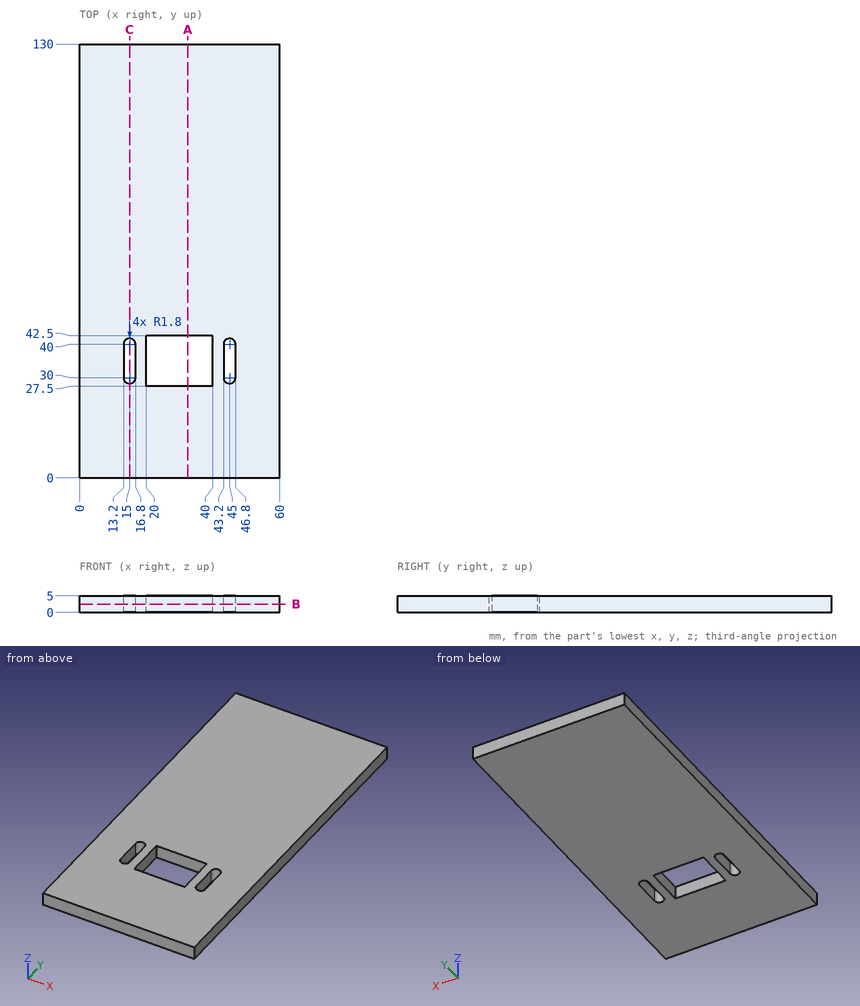
Source: three-view drawing plus pictorial views. Frame: mm from the lowest corner of the part. Give positions to 0.01 mm unless a question says otherwise; leave off trailing zeros. Loops run counter-clockwise (first coordinate to the right, second up) from the corner with the lowest first, then second, coordinate; pieces in that order, holes last.
1) Line query: L1, parallel to X at y = 37, z = 0.25; L2, parallel to Y at x = 31.5, z = 1.2. Output: solid intervals per line, ascending.
A:
L1: x = 0 to 13.2, 16.8 to 20, 40 to 43.2, 46.8 to 60
L2: y = 0 to 27.5, 42.5 to 130
2) Section query C-C on x = 15. Return the cut outline in (y, z).
A:
outline: (0, 0) - (28.2, 0) - (28.2, 5) - (0, 5) - close; (41.8, 0) - (130, 0) - (130, 5) - (41.8, 5) - close
3) Section query A-A on x = 32.5. Return the cut outline in (y, z), and give its area (3 significant figures).
A:
outline: (0, 0) - (27.5, 0) - (27.5, 5) - (0, 5) - close; (42.5, 0) - (130, 0) - (130, 5) - (42.5, 5) - close
area: 575 mm2
4) Section query B-B on z = 2.5. Return the cut outline in (x, y), and give its area (3 significant figures).
A:
outline: (0, 0) - (60, 0) - (60, 130) - (0, 130) - close; hole (13.2, 30) arc R1.8 ccw to (16.8, 30) - (16.8, 40) arc R1.8 ccw to (13.2, 40) - close; hole (20, 27.5) - (40, 27.5) - (40, 42.5) - (20, 42.5) - close; hole (43.2, 30) arc R1.8 ccw to (46.8, 30) - (46.8, 40) arc R1.8 ccw to (43.2, 40) - close
area: 7,410 mm2
